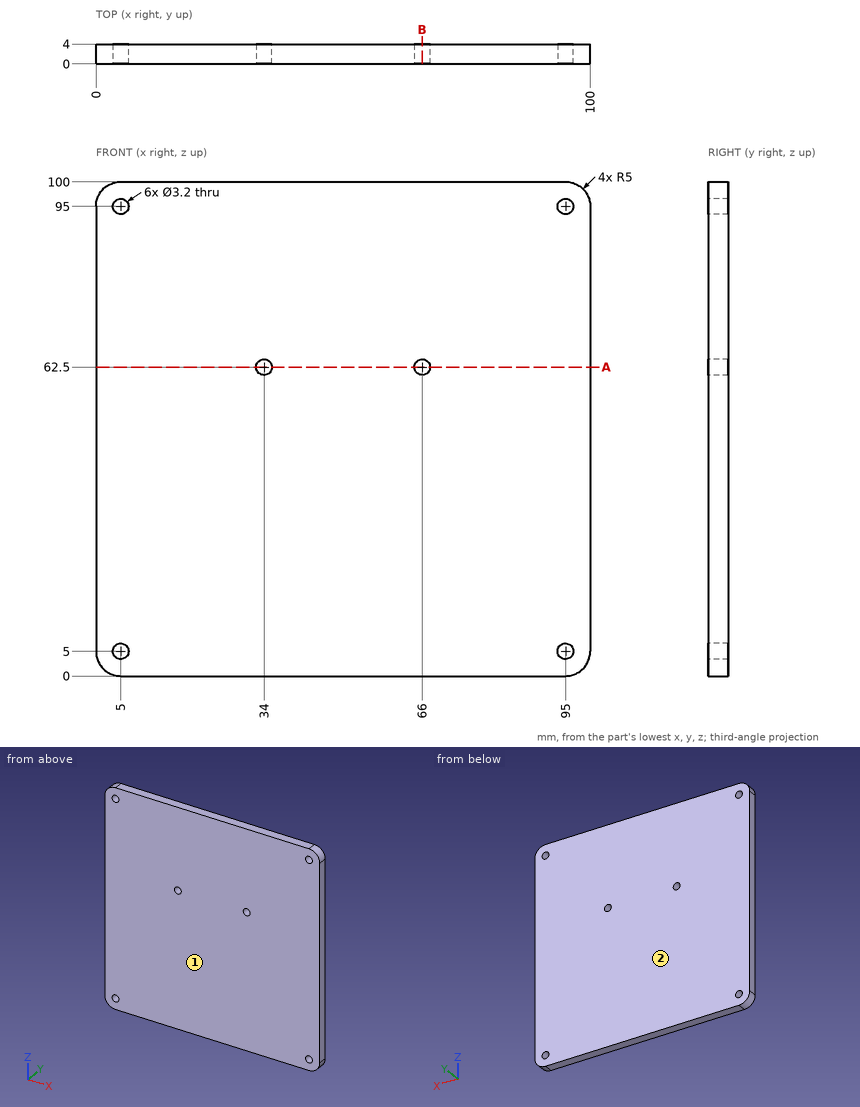
Check sheet for the drawn part. Datum: minimum x, y, z corner. Units: mm. Give positions to 0.01 mm unless a question says otherwise; leave off trailing zeros. Order: outer loops, then holes, each group sorted by start corner. A loop starts at its lowest first (then second) coordinate and runs counter-clockwise, first axis right, second up. Notation, with made-up numbers: (76, 23) -> (84, 23) arc R13 ccw to (84, 44) -> close; hole circle Ø9 at (7, 69). An arc over 180 degrees is marked (long way). One line per item, written item: value.
(1) Gauge pin test, flat end, axial feed: pin 1 (1.9 mm diameter, centred on x = 95, z = 5, fed in from +Y). Record the tip position at first contact, or that the pin passes through.
Final values:
pin 1: through
(2) Sectioned sample at B-B on x = 66. Record the cut outline in (y, z), then the cut area to 3 significant figures.
Final values:
outline: (0, 0) -> (4, 0) -> (4, 60.9) -> (0, 60.9) -> close; (0, 64.1) -> (4, 64.1) -> (4, 100) -> (0, 100) -> close
area: 387 mm^2
(3) Scan lines: line 1 along X through (y, z) = (2.1, 62.5); line 2 along X through (y, z) = (2.25, 5). Record each from-to range of solid material in increasing order. Write a range as [from, to].
Final values:
line 1: [0, 32.4], [35.6, 64.4], [67.6, 100]
line 2: [0, 3.4], [6.6, 93.4], [96.6, 100]
(4) Draft check along Y on the marked faces 1 and 2. Enter one of: pulls with the +Y half, pulls with the -Y half, needs draft (parallel to the pull), parting line crosses it, or undercut.
Final values:
face 1: pulls with the -Y half
face 2: pulls with the +Y half
(5) Sectioned sample at A-A on z = 62.5. Record the cut outline in (x, y), then the cut area to 3 significant figures.
Final values:
outline: (0, 0) -> (32.4, 0) -> (32.4, 4) -> (0, 4) -> close; (35.6, 0) -> (64.4, 0) -> (64.4, 4) -> (35.6, 4) -> close; (67.6, 0) -> (100, 0) -> (100, 4) -> (67.6, 4) -> close
area: 374 mm^2
